Job drawing, mm, ordinate dimensions from the low corner. One solid piece. A direction names the side the tool comes from. Give positions to 0.01 mm unless a question says otherwise; leave off trailing zeros. Loops run counter-clockwise (first coordinate to the right, second up) from the corner with the lowest first, then second, coordinate; pieces in that order, holes last. Notation, with made-up numbers: (79, -28) -> (125, -28) arc R12 ccw to (125, -21) -> close; hole circle Ø10 at (80, -2). An arc over 180 degrees is marked (long way). Answer as a JSON object with one key per item and string values. Group by question number.
Q1. Band-saw the part on D-D, the plane z = 15.5. Write the cut outline in (x, y).
Q2. Band-saw the part on A-A, the plane z = 32. Write the cut outline in (x, y), plus the area to 3 significant figures.
Q3. Band-saw the part on B-B, the plane y = 20.5. Write the cut outline in (x, z).
Q4. Band-saw the part on C-C, the plane x = 35. Write the cut outline in (y, z), plus the area to 3 significant figures.
Q5. Drop flat-ended pins along their axis: pin 1 (4 mm diameter, centred on x = 28.5, z = 5.5, fed in from +Y); pin 2 (12 mm diameter, centred on x = 30, y = 14, fed in from +Z); pin 3 (3.5 mm diameter, centred on x = 35, z = 32, fed in from -Y); pin 4 (0.8 mm diameter, centred on y = 30, z = 0.5, fed in from +X). Give the stop position or say it passes through.
Q6. Tool access for the marked faces 1 and 2: list every direction of +Z, -Z, +X, -X, +Y, -Y with a clear straight run to the whole face (end or side of a thin tool).
Q7. Wall check: probe 1 along X at (y, z) = (0.35, 32); probe 2 along Y at (x, z) = (13, 34). Give the ranges that are in metal, low to high. Write a range as from..to.
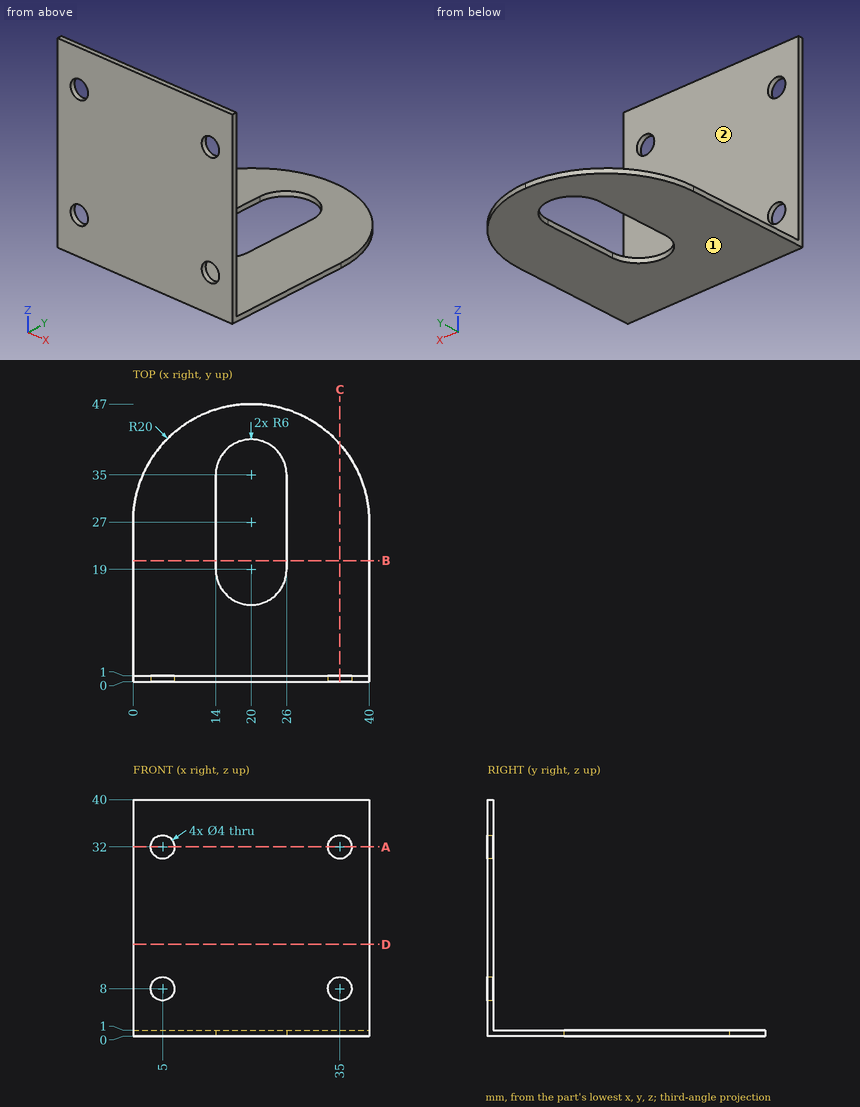
Worked answers:
{
 "1": {"outline": "(0, 0) -> (40, 0) -> (40, 1) -> (0, 1) -> close"},
 "2": {"outline": "(0, 0) -> (3, 0) -> (3, 1) -> (0, 1) -> close; (7, 0) -> (33, 0) -> (33, 1) -> (7, 1) -> close; (37, 0) -> (40, 0) -> (40, 1) -> (37, 1) -> close", "area": "32.0 mm2"},
 "3": {"outline": "(0, 0) -> (14, 0) -> (14, 1) -> (0, 1) -> close; (26, 0) -> (40, 0) -> (40, 1) -> (26, 1) -> close"},
 "4": {"outline": "(0, 0) -> (40.23, 0) -> (40.23, 1) -> (1, 1) -> (1, 6) -> (0, 6) -> close; (0, 10) -> (1, 10) -> (1, 30) -> (0, 30) -> close; (0, 34) -> (1, 34) -> (1, 40) -> (0, 40) -> close", "area": "71.2 mm2"},
 "5": {"pin 1": "y = 1", "pin 2": "z = 1", "pin 3": "through", "pin 4": "x = 39.83"},
 "6": {"face 1": "-Z, +X, -X, +Y, -Y", "face 2": "+Z, +X, -X, +Y"},
 "7": {"probe 1": "0..3, 7..33, 37..40", "probe 2": "0..1"}
}
